```python
from build123d import *

# Parameters (mm, degrees)
F1_DEPTH = 25.4
F3_R     = 24.1381170573
F4_DEPTH = 25.4


# Not quite as in the source:
# - the program builds the solid bodies; features that only make, move or delete a surface that nothing else refers to are left out


with BuildPart() as f1:
    # F0 (on Right) → F1 (new body)
    with BuildSketch(Plane.YZ):
        with BuildLine():
            ThreePointArc((27.3132670653, 48.3872874563), (-47.984242661, -28.0152922777), (55.5638744614, 0))
            ThreePointArc((55.5638744614, 0), (55.2010789182, 6.3391664614), (54.1174299211, 12.5955517503))
            ThreePointArc((54.1174299211, 12.5955517503), (26.1882593397, 19.6121913174), (27.3132670653, 48.3872874563))
        make_face()
        with BuildLine():
            ThreePointArc((27.3132670653, 48.3872874563), (26.1882593397, 19.6121913174), (54.1174299211, 12.5955517503))
            ThreePointArc((54.1174299211, 12.5955517503), (44.4747309057, 33.3067929411), (27.3132670653, 48.3872874563))
        make_face()
        with BuildLine():
            ThreePointArc((27.3132670653, 48.3872874563), (44.4747309057, 33.3067929411), (54.1174299211, 12.5955517503))
            ThreePointArc((54.1174299211, 12.5955517503), (63.739124452, 21.0259013912), (67.3206748777, 33.3067929411))
            ThreePointArc((67.3206748777, 33.3067929411), (52.5328732039, 54.6844330979), (27.3132670653, 48.3872874563))
        make_face()
    extrude(amount=F1_DEPTH)

    # F3 (on face) → F4 (cut)
    with BuildSketch(Plane.YZ.offset(25.4)):
        Circle(F3_R)
    extrude(amount=-F4_DEPTH, mode=Mode.SUBTRACT)


solid = f1.part
```
Model file for the job. Use its own axes, mm. Coordinates: 2 decimals unless noted, no trailing zeros. Order: outer loops, then holes, each group sorted by start corner. A loop starts at its lowest first (then second) coordinate and runs counter-clockwise, first axis right, second up. Notation, with made-up numbers: (45.5, -7.75) -> (103.5, -7.75) arc R22 ccw to (103.5, 0.25) -> close; hole circle Ø9 at (51.25, -18). An arc over 180 degrees is marked (long way). Return JSON: item names as keys, results as strings.
Item 1: Mould opens along Y. For faces 1 (the face through (0, 5, 26)), 2 (the face through (12.878, -5.233, -23.564)) say: pulls with the +Y half, pulls with the -Y half, needs draft (parallel to the pull), parting line crosses it, or undercut.
Model answer:
{"face 1": "needs draft", "face 2": "undercut"}
Item 2: Slice it at C-C (x = 21). Write the cut outline in (y, z), then the cut area to 3 significant figures.
Model answer:
{"outline": "(27.31, 48.39) arc R55.56 ccw (long way) to (54.12, 12.6) arc R22.85 ccw (long way) to start; hole circle Ø48.28 at (0, 0)", "area": "8,760 mm²"}
Item 3: Pin check, flat tips, straight feed: P1, Ø2, axis at x = 4.5, y = 49.5, coming from the +Z side; P2, Ø12, axis at x = 15, y = 33.5, coming from the +Z side; P3, Ø12, axis at x = 12, z = 24, coming from the -Y side. Stop position of each tip, or through.
Model answer:
{"P1": "stops at z = 55.8", "P2": "stops at z = 55.6", "P3": "stops at y = -52.57"}
Item 4: Slice it at B-B (z = 4.5). Write the cut outline in (x, y).
Model answer:
{"outline": "(0, -55.38) -> (25.4, -55.38) -> (25.4, -23.71) -> (0, -23.71) -> close; (0, 23.71) -> (25.4, 23.71) -> (25.4, 55.38) -> (0, 55.38) -> close"}
Item 5: Wall check: line 1 along Z through (x, y) = (16.5, 0); line 2 along Z through (x, y) = (23.5, -7); line 3 along Y through (x, z) = (13, 9). Give the ranges that are in metal, low to high. Write a range as from..to.
Model answer:
{"line 1": "z = -55.56..-24.14, 24.14..55.56", "line 2": "z = -55.12..-23.1, 23.1..55.12", "line 3": "y = -54.83..-22.4, 22.4..54.83"}
Item 6: Slice it at A-A (y = 0). Write the cut outline in (x, z), then the cut area to 3 significant figures.
Model answer:
{"outline": "(0, -55.56) -> (25.4, -55.56) -> (25.4, -24.14) -> (0, -24.14) -> close; (0, 24.14) -> (25.4, 24.14) -> (25.4, 55.56) -> (0, 55.56) -> close", "area": "1,600 mm²"}
Item 7: Slice it at D-D (z = 42.5). Write the cut outline in (x, y), then the cut area to 3 significant figures.
Model answer:
{"outline": "(0, -35.79) -> (25.4, -35.79) -> (25.4, 65.39) -> (0, 65.39) -> close", "area": "2,570 mm²"}
